Model file for the job. Use its own axes, mm. Face numbers are marked on the shaded views. A direction names the side the tool comes from. Give positions to 0.01 mm unless a question says otherwise; leave off trailing zeros. Write each loop counter-clockwise with the first axis right and the second up, starting at its lowest first coordinate (ties: lowest second). Pieces come first, ordered by that corner, then holes. Notation, with made-up numbers: (-14.75, 14.25) - (11.25, 14.25) arc R33 cw to (11.25, 51.25) - close; hole circle Ø8 at (78, 10). An arc over 180 degrees is marked (long way). Use a Markdown table: item, result. Add a question column.
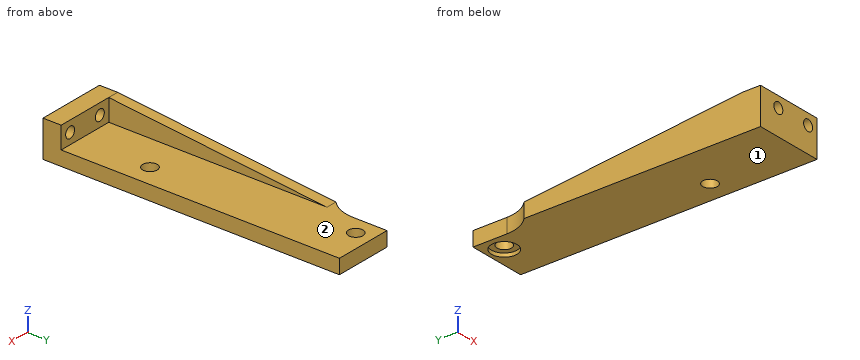
```python
from build123d import *

# Parameters (mm, degrees)
SKETCH_1_W          = 16
SKETCH_1_H          = 6
SKETCH_1_R          = 1.5
EXTRUDE_1_DEPTH     = 5
SKETCH_2_W          = 16
SKETCH_2_H          = 81.5
EXTRUDE_2_DEPTH     = 4
SKETCH_3_R          = 2
CUT_EXTRUDE_1_DEPTH = 83.717894074
SKETCH_4_R          = 2
CUT_EXTRUDE_2_DEPTH = 83.717894074
SKETCH_5_R          = 3.5
CUT_EXTRUDE_3_DEPTH = 1
EXTRUDE_3_DEPTH     = 3
FILLET_1_R          = 10


with BuildPart() as part:
    # 草图1 → 凸台-拉伸1 (new body)
    with BuildSketch(Plane(origin=(0, 0, 0), x_dir=(1, 0, 0), z_dir=(0, 1, 0))):
        with Locations((-2, 0)):
            Rectangle(SKETCH_1_W, SKETCH_1_H)
        with Locations(Location((-7, 0, 0), (0, 0, 270))):
            Circle(SKETCH_1_R, mode=Mode.SUBTRACT)
        with Locations(Location((3, 0, 0), (0, 0, 270))):
            Circle(SKETCH_1_R, mode=Mode.SUBTRACT)
    extrude(amount=EXTRUDE_1_DEPTH)

    # 草图2 → 凸台-拉伸2 (add)
    with BuildSketch(Plane(origin=(0, 0, -3), x_dir=(-1, 0, 0), z_dir=(0, 0, -1))):
        with Locations((2, 40.75)):
            Rectangle(SKETCH_2_W, SKETCH_2_H)
    extrude(amount=EXTRUDE_2_DEPTH)

    # 草图3 → 切除-拉伸1 (cut, through all)
    with BuildSketch(Plane(origin=(0, 0, -7), x_dir=(-1, 0, 0), z_dir=(0, 0, -1))):
        with Locations((5, 77)):
            Circle(SKETCH_3_R)
    extrude(amount=-CUT_EXTRUDE_1_DEPTH, mode=Mode.SUBTRACT)

    # 草图4 → 切除-拉伸2 (cut, through all)
    with BuildSketch(Plane(origin=(0, 0, -7), x_dir=(-1, 0, 0), z_dir=(0, 0, -1))):
        with Locations((0, 24.5)):
            Circle(SKETCH_4_R)
    extrude(amount=-CUT_EXTRUDE_2_DEPTH, mode=Mode.SUBTRACT)

    # 草图5 → 切除-拉伸3 (cut)
    with BuildSketch(Plane(origin=(0, 0, -7), x_dir=(-1, 0, 0), z_dir=(0, 0, -1))):
        with Locations((5, 77)):
            Circle(SKETCH_5_R)
    extrude(amount=-CUT_EXTRUDE_3_DEPTH, mode=Mode.SUBTRACT)

    # 草图6 → 凸台-拉伸3 (add)
    with BuildSketch(Plane.ZY.offset(10)):
        Polygon((3, 5), (-3, 5), (-3, 65), (-7, 65), (-7, 0), (3, 0), align=None)
        Polygon((-3, 65), (-3, 5), (3, 5), align=None)
    extrude(amount=EXTRUDE_3_DEPTH)

    # 圆角1
    # the kernel refuses this fillet: 10 mm, written as the material it adds along each edge
    with BuildSketch(Plane(origin=(-10, 65, -3), x_dir=(-1, 0, 0), z_dir=(0, 0, -1))) as fillet_1_piece_1:
        with BuildLine():
            CenterArc((10, 7.141428429), FILLET_1_R, 180, 45.572995999)
            Line((0, 7.141428429), (0, 0))
            Line((0, 0), (3, 0))
        make_face()
    extrude(amount=4)


solid = part.part
```
(1) Which spindle directions (+Z, -Z, +X, -X, +Y, -Y) get a long thin tool onto all of the face, cutting with end or side? Do the marked faces 1 and 2. Say none if no direction does.
(2) Band-saw the part on D-D (z = -0.25). Write the cut outline in (x, y).
(3) Band-saw the part on C-C (y = 15.5). Write the cut outline in (x, z).
(4) Band-saw the part on B-B (y = 24.5). Write the cut outline in (x, z).
(5) Probe probe 1 along X at (y, z) = (3.9, 0); probe 2 along Y at (x, z) = (-5.25, -4.25); probe 3 along Y at (x, z) = (0, -4.9). List the from-to ranges inside material, lowest first. Write a range as [from, to].
(6) Flat gauge pins, fed straight in: pin 1 (4 mm diameter, centred on x = -5.5, y = 43.5, fed in from +Z); pin 2 (6.5 mm diameter, centred on x = -5, y = 77, fed in from -Z); pin 3 (1.5 mm diameter, centred on x = -5.5, z = 0.5, fed in from +Y). Where does each tip first touch, or does it go through?
(7) Band-saw the part on A-A (z = -5). Write the cut outline in (x, y), then the cut area to 3 significant figures.
Model answer:
| question | item | result |
|---|---|---|
| 1 | face 1 | -Z, +X, -X, +Y, -Y |
| 1 | face 2 | +Z, +X, +Y |
| 2 | outline | (-13, 0) - (-8.48, 0) - (-8.48, 5) - (-10, 5) - (-10, 37.5) - (-13, 37.5) - close; (-5.52, 0) - (1.52, 0) - (1.52, 5) - (-5.52, 5) - close; (4.48, 0) - (6, 0) - (6, 5) - (4.48, 5) - close |
| 3 | outline | (-13, -7) - (6, -7) - (6, -3) - (-10, -3) - (-10, 1.95) - (-13, 1.95) - close |
| 4 | outline | (-13, -7) - (-2, -7) - (-2, -3) - (-10, -3) - (-10, 1.05) - (-13, 1.05) - close; (2, -7) - (6, -7) - (6, -3) - (2, -3) - close |
| 5 | probe 1 | x = [-13, -8.5], [-5.5, 1.5], [4.5, 6] |
| 5 | probe 2 | y = [0, 75.02], [78.98, 81.5] |
| 5 | probe 3 | y = [0, 22.5], [26.5, 81.5] |
| 6 | pin 1 | stops at z = -3 |
| 6 | pin 2 | stops at z = -6 |
| 6 | pin 3 | stops at y = 5 |
| 7 | outline | (-13, 0) - (6, 0) - (6, 81.5) - (-10, 81.5) - (-10, 72.14) arc R10 cw to (-13, 65) - close; hole circle Ø4 at (-5, 77); hole circle Ø4 at (0, 24.5) |
| 7 | area | 1,480 mm^2 |
